Read the model definition and answer for the solid it produces. Units are mm, in the model's axes. Face numbers are marked on the shaded views. Coordinates: 2 decimals unless noted, no trailing zeros. Loops run counter-clockwise (first coordinate to the right, second up) from the corner with the lowest first, then second, coordinate; pieces in that order, holes last.
from build123d import *

# Parameters (mm, degrees)
F1_DEPTH = 3.81
F2_DEPTH = 3.048


with BuildPart() as f1:
    # F0 (on Top) → F1 (new body)
    with BuildSketch(Plane.XY):
        with BuildLine():
            ThreePointArc((-19.510121746, 6.3950662109), (-22.3157867582, 9.0185520845), (-26.0244197252, 10.0187899587))
            Line((-26.0244197252, 10.0187899587), (-26.0244197252, 6.3950662109))
            Line((-26.0244197252, 6.3950662109), (-19.510121746, 6.3950662109))
        make_face()
        with BuildLine():
            Line((-26.0244197252, 6.3950662109), (-26.0244197252, 10.0187899587))
            ThreePointArc((-26.0244197252, 10.0187899587), (-34.1203354035, 2.0770662109), (-26.0244197252, -5.8646575368))
            Line((-26.0244197252, -5.8646575368), (-26.0244197252, -2.2382320992))
            ThreePointArc((-26.0244197252, -2.2382320992), (-30.4951433134, 2.0770662109), (-26.0244197252, 6.3923645211))
            Line((-26.0244197252, 6.3923645211), (-26.0244197252, 6.3950662109))
        make_face()
        with BuildLine():
            Line((37.4916443036, 10.0187899587), (-26.0244197252, 10.0187899587))
            ThreePointArc((-26.0244197252, 10.0187899587), (-22.3157867582, 9.0185520845), (-19.510121746, 6.3950662109))
            Line((-19.510121746, 6.3950662109), (31.1912137245, 6.3950662109))
            ThreePointArc((31.1912137245, 6.3950662109), (33.9031065879, 8.9690226069), (37.4916443036, 10.0187899587))
        make_face()
        with BuildLine():
            Line((38.2424543545, 10.0187899587), (37.4916443036, 10.0187899587))
            ThreePointArc((37.4916443036, 10.0187899587), (33.9031065879, 8.9690226069), (31.1912137245, 6.3950662109))
            Line((31.1912137245, 6.3950662109), (38.2424543545, 6.3950662109))
            Line((38.2424543545, 6.3950662109), (38.2424543545, 10.0187899587))
        make_face()
        with BuildLine():
            ThreePointArc((-19.5083727315, -2.2382320992), (-22.3143805661, -4.8636372504), (-26.0244197252, -5.8646575368))
            Line((-26.0244197252, -5.8646575368), (37.4916443036, -5.8646575368))
            ThreePointArc((37.4916443036, -5.8646575368), (33.9017122748, -4.8140880512), (31.1894670186, -2.2382320992))
            Line((31.1894670186, -2.2382320992), (-19.5083727315, -2.2382320992))
        make_face()
        with BuildLine():
            Line((-26.0244197252, -2.2382320992), (-26.0244197252, -5.8646575368))
            ThreePointArc((-26.0244197252, -5.8646575368), (-22.3143805661, -4.8636372504), (-19.5083727315, -2.2382320992))
            Line((-19.5083727315, -2.2382320992), (-26.0244197252, -2.2382320992))
        make_face()
        with BuildLine():
            ThreePointArc((45.8176408176, 2.0770662109), (43.6201614007, 7.5646527942), (38.2424543545, 10.0187899587))
            Line((38.2424543545, 10.0187899587), (38.2424543545, 6.3950662109))
            ThreePointArc((38.2424543545, 6.3950662109), (41.2957414356, 5.1303532921), (42.5604543545, 2.0770662109))
            ThreePointArc((42.5604543545, 2.0770662109), (41.2957414356, -0.9762208702), (38.2424543545, -2.2409337891))
            Line((38.2424543545, -2.2409337891), (38.2424543545, -5.8646575368))
            ThreePointArc((38.2424543545, -5.8646575368), (43.6201614007, -3.4105203724), (45.8176408176, 2.0770662109))
        make_face()
        with BuildLine():
            ThreePointArc((31.1894670186, -2.2382320992), (33.9017122748, -4.8140880512), (37.4916443036, -5.8646575368))
            Line((37.4916443036, -5.8646575368), (38.2424543545, -5.8646575368))
            Line((38.2424543545, -5.8646575368), (38.2424543545, -2.2409337891))
            ThreePointArc((38.2424543545, -2.2409337891), (38.1660806131, -2.2402583138), (38.0897307663, -2.2382320992))
            Line((38.0897307663, -2.2382320992), (31.1894670186, -2.2382320992))
        make_face()
    extrude(amount=F1_DEPTH)

    # F0 (on Top) → F2 (join)
    with BuildSketch(Plane.XY):
        with BuildLine():
            Line((37.4916443036, 10.0187899587), (-26.0244197252, 10.0187899587))
            ThreePointArc((-26.0244197252, 10.0187899587), (-22.3157867582, 9.0185520845), (-19.510121746, 6.3950662109))
            Line((-19.510121746, 6.3950662109), (31.1912137245, 6.3950662109))
            ThreePointArc((31.1912137245, 6.3950662109), (33.9031065879, 8.9690226069), (37.4916443036, 10.0187899587))
        make_face()
        with BuildLine():
            Line((31.1912137245, 6.3950662109), (-19.510121746, 6.3950662109))
            ThreePointArc((-19.510121746, 6.3950662109), (-18.5596721596, 4.3283844472), (-18.2339512233, 2.0770662109))
            ThreePointArc((-18.2339512233, 2.0770662109), (-18.5592162228, -0.1727087604), (-19.5083727315, -2.2382320992))
            Line((-19.5083727315, -2.2382320992), (31.1894670186, -2.2382320992))
            ThreePointArc((31.1894670186, -2.2382320992), (29.9164580032, 2.0786747903), (31.1912137245, 6.3950662109))
        make_face()
        with BuildLine():
            Line((38.2424543545, 10.0187899587), (37.4916443036, 10.0187899587))
            ThreePointArc((37.4916443036, 10.0187899587), (33.9031065879, 8.9690226069), (31.1912137245, 6.3950662109))
            Line((31.1912137245, 6.3950662109), (38.2424543545, 6.3950662109))
            Line((38.2424543545, 6.3950662109), (38.2424543545, 10.0187899587))
        make_face()
        with BuildLine():
            Line((38.2424543545, 6.3950662109), (31.1912137245, 6.3950662109))
            ThreePointArc((31.1912137245, 6.3950662109), (29.9164580032, 2.0786747903), (31.1894670186, -2.2382320992))
            Line((31.1894670186, -2.2382320992), (38.0897307663, -2.2382320992))
            ThreePointArc((38.0897307663, -2.2382320992), (33.9251298298, 2.1534399524), (38.2424543545, 6.3950662109))
        make_face()
        with BuildLine():
            Line((38.2424543545, -2.2382320992), (38.2424543545, 6.3950662109))
            ThreePointArc((38.2424543545, 6.3950662109), (33.9251298298, 2.1534399524), (38.0897307663, -2.2382320992))
            Line((38.0897307663, -2.2382320992), (38.2424543545, -2.2382320992))
        make_face()
        with BuildLine():
            ThreePointArc((42.5604543545, 2.0770662109), (41.2957414356, 5.1303532921), (38.2424543545, 6.3950662109))
            Line((38.2424543545, 6.3950662109), (38.2424543545, -2.2382320992))
            Line((38.2424543545, -2.2382320992), (38.2424543545, -2.2409337891))
            ThreePointArc((38.2424543545, -2.2409337891), (41.2957414356, -0.9762208702), (42.5604543545, 2.0770662109))
        make_face()
        with BuildLine():
            ThreePointArc((45.8176408176, 2.0770662109), (43.6201614007, 7.5646527942), (38.2424543545, 10.0187899587))
            Line((38.2424543545, 10.0187899587), (38.2424543545, 6.3950662109))
            ThreePointArc((38.2424543545, 6.3950662109), (41.2957414356, 5.1303532921), (42.5604543545, 2.0770662109))
            ThreePointArc((42.5604543545, 2.0770662109), (41.2957414356, -0.9762208702), (38.2424543545, -2.2409337891))
            Line((38.2424543545, -2.2409337891), (38.2424543545, -5.8646575368))
            ThreePointArc((38.2424543545, -5.8646575368), (43.6201614007, -3.4105203724), (45.8176408176, 2.0770662109))
        make_face()
        with BuildLine():
            ThreePointArc((31.1894670186, -2.2382320992), (33.9017122748, -4.8140880512), (37.4916443036, -5.8646575368))
            Line((37.4916443036, -5.8646575368), (38.2424543545, -5.8646575368))
            Line((38.2424543545, -5.8646575368), (38.2424543545, -2.2409337891))
            ThreePointArc((38.2424543545, -2.2409337891), (38.1660806131, -2.2402583138), (38.0897307663, -2.2382320992))
            Line((38.0897307663, -2.2382320992), (31.1894670186, -2.2382320992))
        make_face()
        with BuildLine():
            ThreePointArc((-19.5083727315, -2.2382320992), (-22.3143805661, -4.8636372504), (-26.0244197252, -5.8646575368))
            Line((-26.0244197252, -5.8646575368), (37.4916443036, -5.8646575368))
            ThreePointArc((37.4916443036, -5.8646575368), (33.9017122748, -4.8140880512), (31.1894670186, -2.2382320992))
            Line((31.1894670186, -2.2382320992), (-19.5083727315, -2.2382320992))
        make_face()
        with BuildLine():
            Line((-19.510121746, 6.3950662109), (-26.0244197252, 6.3950662109))
            Line((-26.0244197252, 6.3950662109), (-26.0244197252, 6.3923645211))
            ThreePointArc((-26.0244197252, 6.3923645211), (-23.0703294749, 5.0758712685), (-21.8591433134, 2.0770662109))
            ThreePointArc((-21.8591433134, 2.0770662109), (-23.0703294749, -0.9217388466), (-26.0244197252, -2.2382320992))
            Line((-26.0244197252, -2.2382320992), (-19.5083727315, -2.2382320992))
            ThreePointArc((-19.5083727315, -2.2382320992), (-18.5592162228, -0.1727087604), (-18.2339512233, 2.0770662109))
            ThreePointArc((-18.2339512233, 2.0770662109), (-18.5596721596, 4.3283844472), (-19.510121746, 6.3950662109))
        make_face()
        with BuildLine():
            Line((-26.0244197252, -2.2382320992), (-26.0244197252, 6.3923645211))
            ThreePointArc((-26.0244197252, 6.3923645211), (-30.4951433134, 2.0770662109), (-26.0244197252, -2.2382320992))
        make_face()
        with BuildLine():
            ThreePointArc((-21.8591433134, 2.0770662109), (-23.0703294749, 5.0758712685), (-26.0244197252, 6.3923645211))
            Line((-26.0244197252, 6.3923645211), (-26.0244197252, -2.2382320992))
            ThreePointArc((-26.0244197252, -2.2382320992), (-23.0703294749, -0.9217388466), (-21.8591433134, 2.0770662109))
        make_face()
        with BuildLine():
            ThreePointArc((-19.510121746, 6.3950662109), (-22.3157867582, 9.0185520845), (-26.0244197252, 10.0187899587))
            Line((-26.0244197252, 10.0187899587), (-26.0244197252, 6.3950662109))
            Line((-26.0244197252, 6.3950662109), (-19.510121746, 6.3950662109))
        make_face()
        with BuildLine():
            Line((-26.0244197252, -2.2382320992), (-26.0244197252, -5.8646575368))
            ThreePointArc((-26.0244197252, -5.8646575368), (-22.3143805661, -4.8636372504), (-19.5083727315, -2.2382320992))
            Line((-19.5083727315, -2.2382320992), (-26.0244197252, -2.2382320992))
        make_face()
    extrude(amount=F2_DEPTH)


solid = f1.part
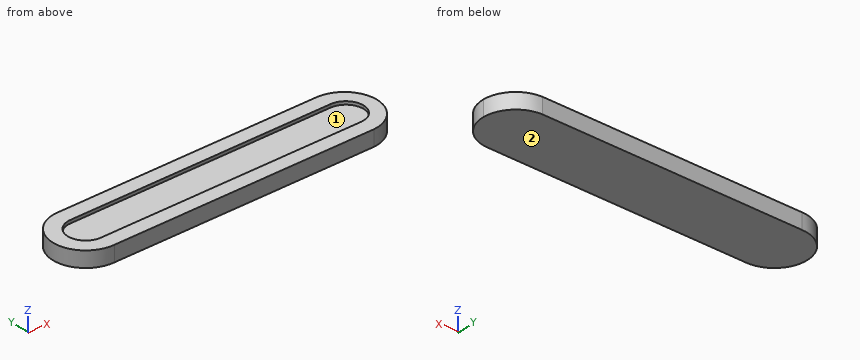
Q1. A flat-ended cylindrical pin translates along its axis: pin 1 Ø2.5 at (x, y) = (22.5, 1.5) entering from +Z. Find the tip coordinate at first contact, or state that the pin passes through.
Findings below:
pin 1: stops at z = 3.05
Q2. Determine the mould class of the marked faces 1 and 2 for opening direction X: +X half, -X half, draft (parallel to the pull), parting line (faces both ways), or undercut.
Findings below:
face 1: undercut
face 2: draft
Q3. A cutting plane is placed at B-B (x = -12.5). Give the vertices of the cut face in (y, z), then the cut area to 3 significant figures.
Findings below:
outline: (-5.86, 0) - (10.02, 0) - (10.02, 3.81) - (6.4, 3.81) - (6.4, 3.05) - (-2.24, 3.05) - (-2.24, 3.81) - (-5.86, 3.81) - close
area: 53.9 mm2
Q4. A cutting plane is placed at D-D (y = 8.75). Give the vertices of the cut face in (x, z).
Findings below:
outline: (-30.49, 0) - (42.19, 0) - (42.19, 3.81) - (-30.49, 3.81) - close
Q5. A cutting plane is placed at C-C (y = 5.5). Give the vertices of the cut face in (x, z), then the cut area to 3 significant figures.
Findings below:
outline: (-33.34, 0) - (45.04, 0) - (45.04, 3.81) - (40.87, 3.81) - (40.87, 3.05) - (-28.81, 3.05) - (-28.81, 3.81) - (-33.34, 3.81) - close
area: 246 mm2
Q6. Straight lines are drawn through the part: probe 1 along Z at (x, y) = (36.5, 2.5); probe 2 along Y at (x, z) = (-6, 0.95); probe 3 along Y at (x, z) = (8.5, 3.65). For each, find the intervals that lie inside material, in ascending order.
Findings below:
probe 1: z = 0 to 3.05
probe 2: y = -5.86 to 10.02
probe 3: y = -5.86 to -2.24, 6.4 to 10.02
